```python
from build123d import *

# Parameters (mm, degrees)
ESQUISSE1_W           = 60
ESQUISSE1_H           = 65
BOSS_EXTRU_1_DEPTH    = 12
TROU_TARAUD_M57_D     = 4.2
TROU_TARAUD_M57_DEPTH = 14
TROU_TARAUD_M57_TIP   = 1.2618073
TROU_TARAUD_M58_D     = 4.2
TROU_TARAUD_M58_DEPTH = 14
TROU_TARAUD_M58_TIP   = 1.2618073
TROU_TARAUD_M56_D     = 4.2
TROU_TARAUD_M56_DEPTH = 14
TROU_TARAUD_M56_TIP   = 1.2618073
TROU_TARAUD_M55_D     = 4.2
TROU_TARAUD_M55_DEPTH = 14
TROU_TARAUD_M55_TIP   = 1.2618073


with BuildPart() as part:
    # Esquisse1 → Boss.-Extru.1 (new body)
    with BuildSketch(Plane.XY):
        with Locations((30, 32.5)):
            Rectangle(ESQUISSE1_W, ESQUISSE1_H)
    extrude(amount=BOSS_EXTRU_1_DEPTH)

    # Trou taraudé M57
    with Locations(Plane(origin=(0, 65, 0), x_dir=(-1, 0, 0), z_dir=(0, 1, 0))):
        with Locations((-8, 6)):
            Hole(TROU_TARAUD_M57_D / 2, depth=TROU_TARAUD_M57_DEPTH)
            with Locations((0, 0, -(TROU_TARAUD_M57_DEPTH + TROU_TARAUD_M57_TIP / 2))):  # 118° drill point
                Cone(0, TROU_TARAUD_M57_D / 2, TROU_TARAUD_M57_TIP, mode=Mode.SUBTRACT)

    # Trou taraudé M58
    with Locations(Plane(origin=(0, 65, 0), x_dir=(-1, 0, 0), z_dir=(0, 1, 0))):
        with Locations((-52, 6)):
            Hole(TROU_TARAUD_M58_D / 2, depth=TROU_TARAUD_M58_DEPTH)
            with Locations((0, 0, -(TROU_TARAUD_M58_DEPTH + TROU_TARAUD_M58_TIP / 2))):  # 118° drill point
                Cone(0, TROU_TARAUD_M58_D / 2, TROU_TARAUD_M58_TIP, mode=Mode.SUBTRACT)

    # Trou taraudé M56
    with Locations(Plane.XZ):
        with Locations((8, 6)):
            Hole(TROU_TARAUD_M56_D / 2, depth=TROU_TARAUD_M56_DEPTH)
            with Locations((0, 0, -(TROU_TARAUD_M56_DEPTH + TROU_TARAUD_M56_TIP / 2))):  # 118° drill point
                Cone(0, TROU_TARAUD_M56_D / 2, TROU_TARAUD_M56_TIP, mode=Mode.SUBTRACT)

    # Trou taraudé M55
    with Locations(Plane.XZ):
        with Locations((52, 6)):
            Hole(TROU_TARAUD_M55_D / 2, depth=TROU_TARAUD_M55_DEPTH)
            with Locations((0, 0, -(TROU_TARAUD_M55_DEPTH + TROU_TARAUD_M55_TIP / 2))):  # 118° drill point
                Cone(0, TROU_TARAUD_M55_D / 2, TROU_TARAUD_M55_TIP, mode=Mode.SUBTRACT)


solid = part.part
```
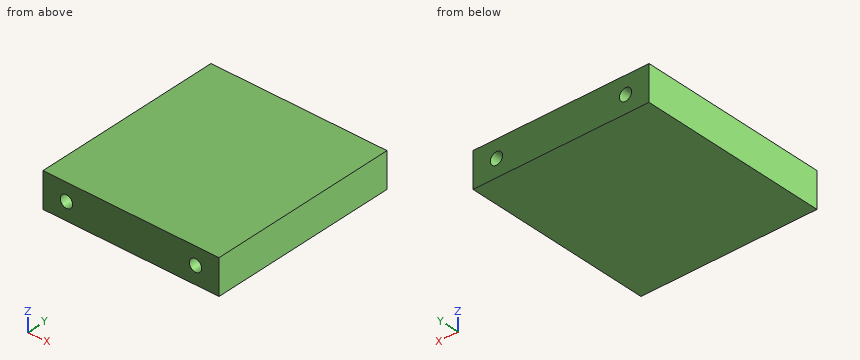
Source: CAD feature listing. Evaluate the final solid. Frame: model axes, mm. Round coordinates to 2 decimals unless told otherwise and drop trailing zeros. Order: outer loops, then holes, each group sorted by start corner. A loop starts at its lowest first (then second) coordinate and runs counter-clockwise, first axis right, second up. Notation, with made-up numbers: (-36.5, -26) -> (1.5, -26) arc R21 cw to (1.5, -12) -> close; hole circle Ø1 at (34, 81.5). An arc over 180 degrees is marked (long way). Use CSV: the item, a comma, the result in double quotes.
(1) Ray query, L1, parallel to X at y = 11.25, z = 6; L2, parallel to Z at x = 8, y = 6.5; L3, parallel to X at y = 4, z = 4.25. Return the intervals inside material, ascending.
Report:
L1,"0 to 5.9, 10.1 to 49.9, 54.1 to 60"
L2,"0 to 3.9, 8.1 to 12"
L3,"0 to 6.84, 9.16 to 50.84, 53.16 to 60"
(2) Section A-A on y = 11. Return the cut outline in (x, z), and give its area (3 significant figures).
Report:
outline,"(0, 0) -> (60, 0) -> (60, 12) -> (0, 12) -> close; hole circle Ø4.2 at (8, 6); hole circle Ø4.2 at (52, 6)"
area,"692 mm^2"
(3) First-contact query: pin 1 Ø2.5 at (x, z) = (52, 6) entering from -Y; pin 2 Ø3.5 at (x, z) = (8, 6) entering from +Y; pin 3 Ø2.5 at (x, z) = (8, 6) entering from +Y. Flat tips, straight axial feed; report the tip coordinate or a pass-through.
Report:
pin 1,"y = 14.51"
pin 2,"y = 50.79"
pin 3,"y = 50.49"
